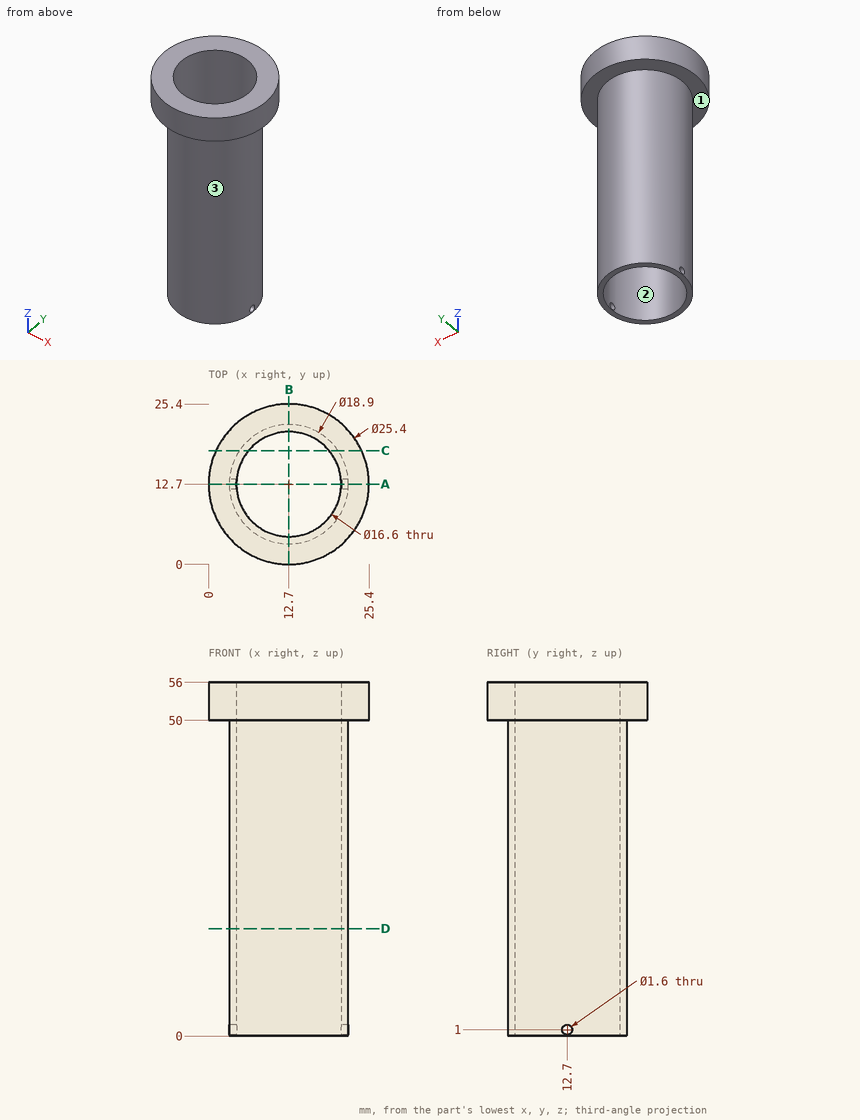
Here's the drawing with two shaded views (mm, measured from the low corner). I have some questions. Give positions to 0.01 mm unless a question says otherwise; leave off trailing zeros. Loops run counter-clockwise (first coordinate to the right, second up) from the corner with the lowest first, then second, coordinate; pieces in that order, holes last. Notation, with made-up numbers: M 45,12 L 53,12 A24 cw 53,43 Z; hole C 57,2 d1. An arc over 180 degrees is marked long. One line per item, written item: value.
(1) We'd pull the mould along X, two halves only. Please class the marked faces 1, 2 and 3: released by +X, released by -X, zero draft, split by the parting line, or undercut.
Returned:
face 1: zero draft
face 2: undercut
face 3: split by the parting line
(2) Suppose I cut it at A-A on y = 12.7. List the corners of the cut face in (x, z) for me.
Returned:
outline: M 0,50 L 3.25,50 L 3.25,1.8 L 4.4,1.8 L 4.4,56 L 0,56 Z; M 3.25,0 L 4.4,0 L 4.4,0.2 L 3.25,0.2 Z; M 21,0 L 22.15,0 L 22.15,0.2 L 21,0.2 Z; M 21,1.8 L 22.15,1.8 L 22.15,50 L 25.4,50 L 25.4,56 L 21,56 Z
(3) Will these pins go through, and if not, where does the flat tip stop? pin 1 (5 mm diameter, centred on x = 4, z = 25.5, fed in from +Y); pin 2 (10 mm diameter, centred on y = 15, z = 13.5, fed in from +X); pin 3 (6 mm diameter, centred on x = 8.5, z = 29.5, fed in from -Y); pin 4 (1.4 mm diameter, centred on y = 12.7, z = 1, fed in from -X).
Returned:
pin 1: y = 19.83
pin 2: x = 22.15
pin 3: y = 3.33
pin 4: through
(4) Suppose I cut it at D-D on z = 17. List the corners of the cut face in (x, y) for me, plus the area to 3 significant figures.
Returned:
outline: C 12.7,12.7 d18.9; hole C 12.7,12.7 d16.6
area: 64.1 mm^2
(5) I need wall thicknesses on line 1 (Y direction, x = 12.7, z = 38); line 2 (X direction, y = 12.75, z = 54). Which ranges of each line are inside material? Lowest first, please.
Returned:
line 1: 3.25 to 4.4, 21 to 22.15
line 2: 0 to 4.4, 21 to 25.4
(6) Suppose I cut it at C-C on y = 18. List the corners of the cut face in (x, z) for me, plus the area to 3 significant figures.
Returned:
outline: M 1.16,50 L 4.88,50 L 4.88,0 L 6.31,0 L 6.31,56 L 1.16,56 Z; M 19.09,0 L 20.52,0 L 20.52,50 L 24.24,50 L 24.24,56 L 19.09,56 Z
area: 205 mm^2
(7) Suppose I cut it at B-B on x = 12.7. List the corners of the cut face in (y, z) for me, plus the area to 3 significant figures.
Returned:
outline: M 0,50 L 3.25,50 L 3.25,0 L 4.4,0 L 4.4,56 L 0,56 Z; M 21,0 L 22.15,0 L 22.15,50 L 25.4,50 L 25.4,56 L 21,56 Z
area: 168 mm^2
